CAD build for the part. Positions are in the model's coordinates, mm. Face numbers are marked on the shaded views. Coordinates: 2 decimals unless noted, no trailing zeros. Write each loop counter-clockwise with the first axis right and the second up, starting at its lowest first coordinate (ties: lowest second). Pieces come first, ordered by that corner, then holes. Notation, with made-up numbers: (6, -16) -> (63, -16) arc R8 ccw to (63, -1) -> close; hole circle Ø2 at (81, 81). An arc over 180 degrees is marked (long way). Answer as CSV lines item,"result".
```python
from build123d import *

# Parameters (mm, degrees)
F0_R     = 6.544333
F0_R_2   = 6.5405
F1_DEPTH = 25.4
F2_DEPTH = 25.4


with BuildPart() as f1:
    # F0 (on Front) → F1 (new body)
    with BuildSketch(Plane.XZ):
        Polygon((28.962216, 3.225733), (-21.037417, 3.034164), (-21.037417, -16.774267), (28.962216, -16.774267), align=None)
        with Locations((-8.991601, -7.9248)):
            Circle(F0_R, mode=Mode.SUBTRACT)
        with Locations((16.611602, -6.7056)):
            Circle(F0_R_2, mode=Mode.SUBTRACT)
    extrude(amount=F1_DEPTH)

    # F0 (on Front) → F2 (join)
    with BuildSketch(Plane.XZ):
        Polygon((28.962216, 3.225733), (-21.037417, 3.034164), (-21.037417, -16.774267), (28.962216, -16.774267), align=None)
        with Locations((-8.991601, -7.9248)):
            Circle(F0_R, mode=Mode.SUBTRACT)
        with Locations((16.611602, -6.7056)):
            Circle(F0_R_2, mode=Mode.SUBTRACT)
    extrude(amount=F2_DEPTH)


solid = f1.part
```
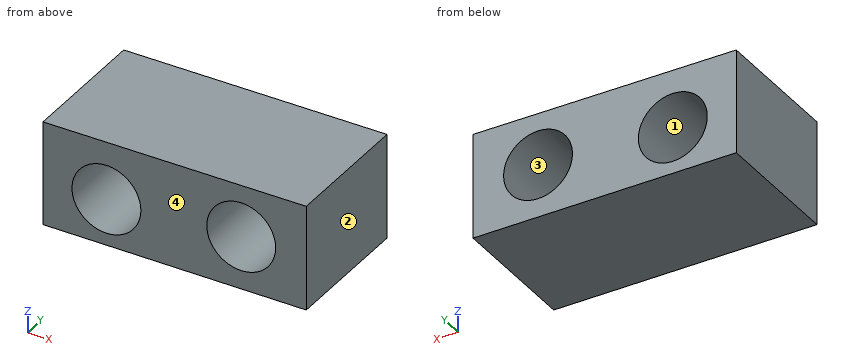
Item 1: Saw through at B-B on x = -6.5. Give the cut face in (y, z).
Answer below:
outline,"(-25.4, -16.77) -> (0, -16.77) -> (0, -13.98) -> (-25.4, -13.98) -> close; (-25.4, -1.87) -> (0, -1.87) -> (0, 3.09) -> (-25.4, 3.09) -> close"
Item 2: Saw through at A-A on z = -12.25. Give the cut face in (x, y), and give its area (3 significant figures).
Answer below:
outline,"(-21.04, -25.4) -> (-13.9, -25.4) -> (-13.9, 0) -> (-21.04, 0) -> close; (-4.08, -25.4) -> (13.14, -25.4) -> (13.14, 0) -> (-4.08, 0) -> close; (20.08, -25.4) -> (28.96, -25.4) -> (28.96, 0) -> (20.08, 0) -> close"
area,"844 mm2"
Item 3: Wall check: line 1 (X direction, y = -8.25, z = -8.25); line 2 (X direction, y = -24.5, z = -4); line 3 (Z direction, x = -8, y = -19.75). Give the ranges that are in metal, low to high. Write a range as from..to.
Answer below:
line 1,"x = -21.04..-15.53, -2.46..10.26, 22.97..28.96"
line 2,"x = -21.04..-14.23, -3.75..10.66, 22.57..28.96"
line 3,"z = -16.77..-14.39, -1.46..3.08"
Item 4: Saw through at C-C on y = -17. Give the cut face in (x, z), and give its area (3 significant figures).
Answer below:
outline,"(-21.04, -16.77) -> (28.96, -16.77) -> (28.96, 3.23) -> (-21.04, 3.03) -> close; hole circle Ø13.09 at (-8.99, -7.92); hole circle Ø13.08 at (16.61, -6.71)"
area,"726 mm2"
Item 5: Saw through at D-D on z = -4. Give the cut face in (x, y).
Answer below:
outline,"(-21.04, -25.4) -> (-14.23, -25.4) -> (-14.23, 0) -> (-21.04, 0) -> close; (-3.75, -25.4) -> (10.66, -25.4) -> (10.66, 0) -> (-3.75, 0) -> close; (22.57, -25.4) -> (28.96, -25.4) -> (28.96, 0) -> (22.57, 0) -> close"
Item 6: Flat gauge pins, fed straight in: pin 1 (5 mm diameter, centred on x = 18.5, y = -16, fed in from +Z); pin 2 (12 mm diameter, centred on x = -8.99, z = -7.92, fed in from +Y); pin 3 (10 mm diameter, centred on x = 4, y = -18, fed in from +Z). Where does each tip first touch, or does it go through?
Answer below:
pin 1,"stops at z = 3.2"
pin 2,"passes through"
pin 3,"stops at z = 3.15"
Item 7: Two-plate mould, pull along X, no slides. Class the marked faces 1, 2, 3 and 4: pulls with the +X half, pulls with the -X half, needs draft (parallel to the pull), parting line crosses it, or undercut.
Answer below:
face 1,"undercut"
face 2,"pulls with the +X half"
face 3,"undercut"
face 4,"needs draft"
